Verification items for the finished model (mm, model axes). A direction names the side the tool comes from. Round coordinates to 2 decimals unless told otherwise and drop trailing zeros. Order: outer loops, then holes, each group sorted by start corner. A loop starts at its lowest first (then second) coordinate and runs counter-clockwise, first axis right, second up. Notation, with made-up numbers: (-22, -3.75) -> (-11, -3.75) arc R14 cw to (-11, 1.25) -> close; hole circle Ø3 at (-1, -12). An arc over 180 degrees is marked (long way). Return JSON: item names as keys, results as strings. Group by question number.
Item 1: Scan lines: probe 1 along Z at (x, y) = (68, 8.5); probe 2 along Z at (x, y) = (126, -9.5); probe 3 along Y at (x, z) = (90, 0.5). Record each from-to range of solid material in increasing order. Write a range as from..to.
Item 2: Access from +Z, -Z, +X, -X, +Y, -Y to the whole of each face (thin tool, end or side, straight path). Record for faces 1 (the flat face through (0, 0, -1)), 2 (the cylindrical face through (25.756, -4.754, 10.195)).
Item 3: Depth check by flat-ended pin: pin 1 Ø6 at (x, z) = (80.5, 4.5) entering from +Y; pin 2 Ø12 at (x, z) = (124.5, 1) entering from +Y; pin 3 Ø12 at (x, y) = (143, 15.5) entering from +Z; pin 4 Ø4 at (x, z) = (109.5, 28) entering from +Y. Enter the tip coordinate at first touch or a pass-through.
Item 4: Sectioned sample at A-A on x = 12. Record the cut outline in (y, z).
```python
from build123d import *

# Parameters (mm, degrees)
SKETCH2_R           = 49.53
BOSS_EXTRUDE1_DEPTH = 203.2
SKETCH3_R           = 12.411567775
BOSS_EXTRUDE2_DEPTH = 50.8
SKETCH4_R           = 49.53
CUT_EXTRUDE1_DEPTH  = 381
SKETCH5_R           = 49.53
CUT_EXTRUDE2_DEPTH  = 381


with BuildPart() as part:
    # Sketch1 → Revolve2 (revolve)
    with BuildSketch(Plane(origin=(0, 0, 0), x_dir=(1, 0, 0), z_dir=(0, 1, 0))):
        with BuildLine():
            Line((355.600000053, 50.799999973), (355.600000053, 1.269999973))
            Line((355.600000053, 1.269999973), (50.800000047, 1.269999973))
            Line((50.800000047, 1.269999973), (50.800000047, 13.68156774))
            add(Edge.make_bspline(
                [(50.800000047, 13.68156774), (51.224607869, 13.786541703), (52.079748124, 13.99736018), (53.901316113, 14.445024847), (55.90428978, 14.933081433), (57.918204029, 15.420277853), (59.969167456, 15.913068852), (62.005618607, 16.398707152), (64.04585603, 16.881716673), (66.619566178, 17.486536085), (69.727395203, 18.209576077), (73.370678613, 19.04644661), (77.55044141, 19.991710093), (82.779136229, 21.155661521), (97.433989811, 24.348822924), (119.485629173, 28.81699746), (168.00075752, 37.516041455), (219.035004801, 44.081341124), (262.822405655, 47.820230422), (299.206459448, 49.570692635), (308.841173655, 49.947366018), (315.265578413, 50.162354186), (319.548981494, 50.29122703), (323.832782669, 50.405645805), (328.116966628, 50.505609209), (332.401425999, 50.591116104), (336.139078075, 50.653092889), (339.329601827, 50.697064227), (341.973247658, 50.727612371), (344.069774299, 50.748376802), (346.163273231, 50.76568058), (348.272494467, 50.77952366), (350.344714481, 50.789906003), (352.405704949, 50.79682758), (354.282013928, 50.799423175), (355.162608625, 50.799999974), (355.600000053, 50.799999973)],
                knots=[0.08282658, 0.08282658, 0.08282658, 0.08282658, 0.08282658, 0.088510594, 0.094194608, 0.099878623, 0.105562637, 0.111246651, 0.116930666, 0.12261468, 0.128298694, 0.139917182, 0.15153567, 0.163154157, 0.174772645, 0.198009616, 0.314194483, 0.407142375, 0.709223026, 0.755696971, 0.790552431, 0.802170918, 0.813789405, 0.825407891, 0.837026378, 0.848644864, 0.860263351, 0.871881838, 0.877565852, 0.883249866, 0.88893388, 0.894617894, 0.900301908, 0.905985922, 0.911669936, 0.91735395, 0.91735395, 0.91735395, 0.91735395, 0.91735395], degree=4))
        make_face()
    revolve(axis=Axis((355.600000053, 0, -1.269999973), (-1, 0, 0)))

    # Sketch2 → Boss-Extrude1 (add)
    with BuildSketch(Plane(origin=(355.600000053, 0, 0), x_dir=(0, 0, -1), z_dir=(1, 0, 0))):
        with Locations((1.269999973, 0)):
            Circle(SKETCH2_R)
    extrude(amount=BOSS_EXTRUDE1_DEPTH)

    # Sketch3 → Boss-Extrude2 (add)
    with BuildSketch(Plane.ZY.offset(-50.800000063)):
        with Locations((-1.269999973, 0)):
            Circle(SKETCH3_R)
    extrude(amount=BOSS_EXTRUDE2_DEPTH)

    # Sketch4 → Cut-Extrude1 (cut)
    with BuildSketch(Plane(origin=(368.300000053, 0, 0), x_dir=(0, 0, -1), z_dir=(1, 0, 0))):
        with Locations((1.269999973, 0)):
            Circle(SKETCH4_R)
    extrude(amount=CUT_EXTRUDE1_DEPTH, mode=Mode.SUBTRACT)

    # Sketch5 → Cut-Extrude2 (cut)
    with BuildSketch(Plane(origin=(177.800000053, 0, 0), x_dir=(0, 0, -1), z_dir=(1, 0, 0))):
        with Locations((1.269999973, 0)):
            Circle(SKETCH5_R)
    extrude(amount=CUT_EXTRUDE2_DEPTH, mode=Mode.SUBTRACT)


solid = part.part
```
Recorded:
{
 "1": {"probe 1": "-15.46..12.92", "probe 2": "-28.25..25.71", "probe 3": "-21.37..21.37"},
 "2": {"face 1": "+Z, -Z, -X, +Y, -Y", "face 2": "-X"},
 "3": {"pin 1": "y = 19.51", "pin 2": "y = 29.38", "pin 3": "z = 29.15", "pin 4": "through"},
 "4": {"outline": "circle Ø24.82 at (0, -1.27)"}
}
